Job drawing, mm, ordinate dimensions from the low corner. One solid piece. A direction names the side the tool comes from. Round coordinates to 2 decimals unless told otherwise and drop trailing zeros. Loops run counter-clockwise (first coordinate to the right, second up) from the corner with the lowest first, then second, coordinate; pieces in that order, holes last. Notation, with made-up numbers: M 10,6 L 14,6 A37 cw 14,42 Z; hole C -26,34.25 d7. An arc over 180 degrees is marked long. Use a Markdown table: item, result. Add a question column.
(1) Two-plate mould, pull along Z, no slides. Class the marked faces 4, 5, 6 and 7: released by +Z, released by -Z, zero draft, split by the parting line, or undercut.
(2) Wall check: L1, parallel to X at y = 1.6, z = 6.25; L2, parallel to Z at x = 3, y = 1.1; L3, parallel to Y at x = 2, z = 9.25. Give the ranges that are in metal, low to high.
(3) Which spindle directions (+Z, -Z, +X, -X, +Y, -Y) get a long thin tool onto all of the face, cutting with end or side? Do the marked faces 1, 2 and 3. Say none if no direction does.
(4) Band-saw the part on D-D, the plane x = 3.5. Write the cut outline in (y, z) (1 decimal).
(5) Band-saw the part on C-C, the plane y = 2.3. Write the cut outline in (x, z).
(6) Band-saw the part on A-A, the plane z = 4.5. Write the cut outline in (x, y).
(7) Flat gauge pins, fed straight in: P1, Ø1, axis at x = 2, z = 7, coming from the +Y side; P2, Ø0.8, axis at x = 3, z = 1, coming from the -Y side; P3, Ø1.5, axis at x = 1.5, y = 2, coming from the +Z side. Where does each tip first touch, or does it go through?
(8) Band-saw the part on B-B, the plane x = 2. Write the cut outline in (y, z).
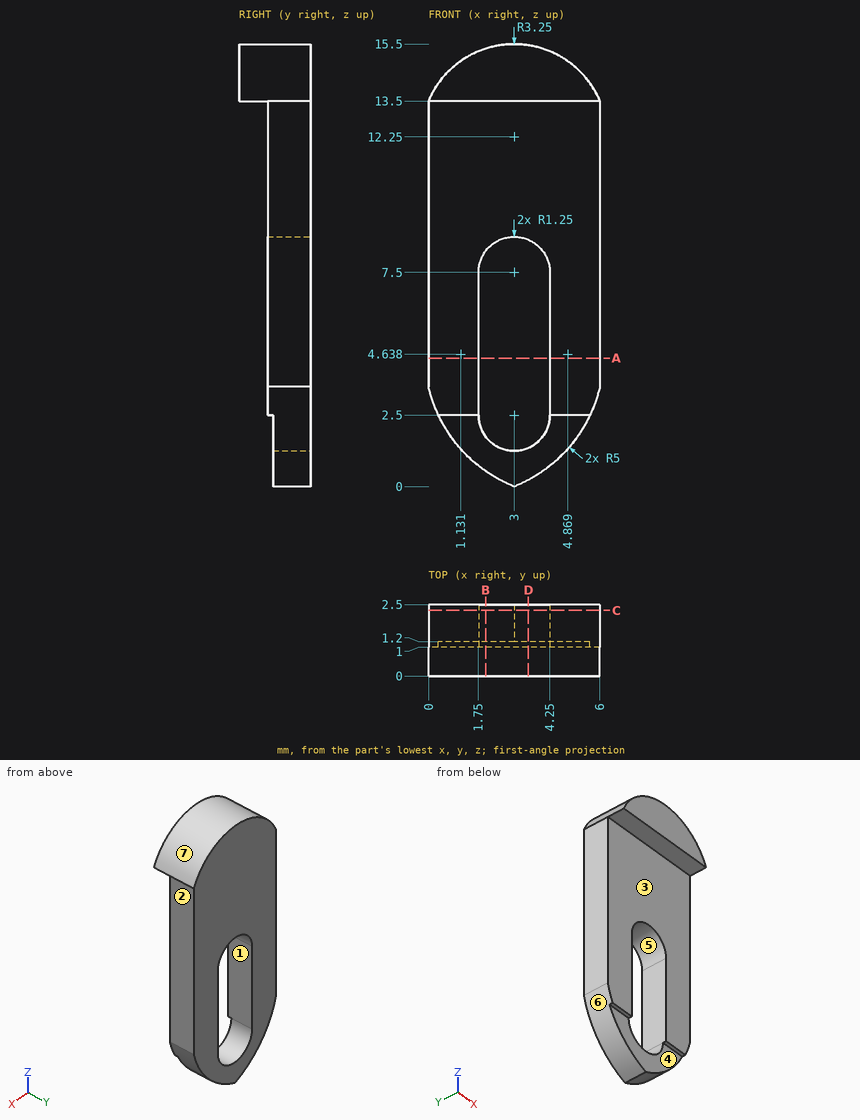
Return value:
| question | item | result |
|---|---|---|
| 1 | face 4 | zero draft |
| 1 | face 5 | undercut |
| 1 | face 6 | released by -Z |
| 1 | face 7 | released by +Z |
| 2 | L1 | 0 to 1.75, 4.25 to 6 |
| 2 | L2 | 8.75 to 15.5 |
| 2 | L3 | 1 to 2.5 |
| 3 | face 1 | +Y, -Y |
| 3 | face 2 | +Z, -Z, +X, +Y, -Y |
| 3 | face 3 | -Z, +X, -X, -Y |
| 4 | outline | M 0,13.5 L 1,13.5 L 1,8.6 L 2.5,8.6 L 2.5,15.5 L 0,15.5 Z; M 1.2,0.2 L 2.5,0.2 L 2.5,1.4 L 1.2,1.4 Z |
| 5 | outline | M 0,3.5 A5 ccw 3,0 A5 ccw 6,3.5 L 6,13.5 A3.25 ccw 0,13.5 Z; hole M 1.75,2.5 A1.25 ccw 4.25,2.5 L 4.25,7.5 A1.25 ccw 1.75,7.5 Z |
| 6 | outline | M 0,1 L 1.75,1 L 1.75,2.5 L 0,2.5 Z; M 4.25,1 L 6,1 L 6,2.5 L 4.25,2.5 Z |
| 7 | P1 | y = 2.5 |
| 7 | P2 | y = 1.2 |
| 7 | P3 | z = 15.41 |
| 8 | outline | M 0,13.5 L 1,13.5 L 1,8.25 L 2.5,8.25 L 2.5,15.34 L 0,15.34 Z; M 1.2,0.54 L 2.5,0.54 L 2.5,1.75 L 1.2,1.75 Z |
